Model file for the job. Use its own axes, mm. Face numbers are marked on the shaded views. A direction names the side the tool comes from. Give positions to 0.01 mm unless a question says otherwise; leave off trailing zeros. Loops run counter-clockwise (first coordinate to the right, second up) from the corner with the lowest first, then second, coordinate; pieces in that order, holes last. Notation, with made-up numbers: (-21, 4.25) - (13, 4.25) arc R17 ccw to (13, 9.25) - close; hole circle Ø8 at (8.25, -10). An arc over 180 degrees is marked (long way). Use a Markdown table: item, result.
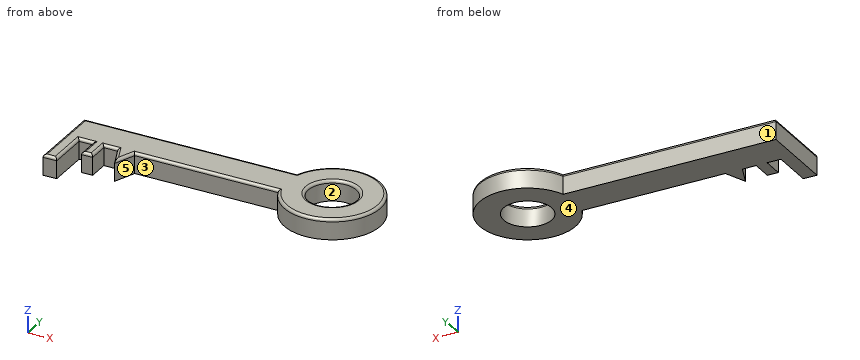
from build123d import *

# Parameters (mm, degrees)
F0_R     = 17.5
F0_W     = 10
F0_H     = 30
F0_W_2   = 8
F0_H_2   = 15
F1_DEPTH = 15
F2_R     = 2


with BuildPart() as f1:
    # F0 (on Top) → F1 (new body)
    with BuildSketch(Plane.XY):
        Polygon((70.049999, 32.850001), (-84.950001, 32.850001), (-84.950001, 7.850001), (-74.950001, 7.850001), (-64.950001, 7.850001), (-56.950001, 7.850001), (-46.950001, 7.850001), (-34.520773, 7.850001), (70.049999, 7.850001), align=None)
        with BuildLine():
            ThreePointArc((70.049999, 7.850001), (137.741741, 20.350001), (70.049999, 32.850001))
            Line((70.049999, 32.850001), (70.049999, 7.850001))
        make_face()
        with Locations((102.741741, 20.350001)):
            Circle(F0_R, mode=Mode.SUBTRACT)
        with Locations((-79.950001, -7.149999)):
            Rectangle(F0_W, F0_H)
        Polygon((-40.735387, -7.49211), (-34.520773, 7.850001), (-46.950001, 7.850001), align=None)
        with Locations((-60.950001, 0.350001)):
            Rectangle(F0_W_2, F0_H_2)
    extrude(amount=F1_DEPTH)

    # F2
    f2_edges = [f1.edges().sort_by_distance(p)[0] for p in [
        (-7.450001, 32.850001, 15),
        (-84.950001, 5.350001, 15),
        (-79.950001, -22.149999, 15),
        (-74.950001, -7.149999, 15),
        (-69.950001, 7.850001, 15),
        (-64.950001, 0.350001, 15),
        (-60.950001, -7.149999, 15),
        (-56.950001, 0.350001, 15),
        (-51.950001, 7.850001, 15),
        (-43.842694, 0.178945, 15),
        (-37.62808, 0.178945, 15),
        (17.764613, 7.850001, 15),
        (137.741741, 20.350001, 15),
        (85.241741, 20.350001, 15),
    ]]
    fillet(f2_edges, radius=F2_R)


solid = f1.part
(1) Slice it at A-A, the plane z = 8.5. Write the cut outline in (x, y).
Computed:
| item | result |
|---|---|
| outline | (-84.95, -22.15) - (-74.95, -22.15) - (-74.95, 7.85) - (-64.95, 7.85) - (-64.95, -7.15) - (-56.95, -7.15) - (-56.95, 7.85) - (-46.95, 7.85) - (-40.74, -7.49) - (-34.52, 7.85) - (70.05, 7.85) arc R35 ccw (long way) to (70.05, 32.85) - (-84.95, 32.85) - close; hole circle Ø35 at (102.74, 20.35) |
(2) Mould opens along X. For the marked faces 1, 2 and 3 say: pulls with the +X half, pulls with the -X half, needs draft (parallel to the pull), parting line crosses it, or undercut.
Computed:
| item | result |
|---|---|
| face 1 | needs draft |
| face 2 | undercut |
| face 3 | undercut |
(3) Slice it at B-B, the plane x = 34. Write the cut outline in (y, z).
Computed:
| item | result |
|---|---|
| outline | (7.85, 0) - (32.85, 0) - (32.85, 13) arc R2 ccw to (30.85, 15) - (9.85, 15) arc R2 ccw to (7.85, 13) - close |
(4) Pin check, flat tips, straight feed: P1, Ø1.5, axis at x = 89, z = 11.5, coming from the -Y side; P2, Ø5, axis at x = -71, z = 8.5, coming from the -Y side; P3, Ø2.5, axis at x = -62, z = 8, coming from the -Y side; P4, Ø21, axis at x = 102.74, y = 20.35, coming from the +Z side. Stop position of each tip, or through.
Computed:
| item | result |
|---|---|
| P1 | y = -12.15 |
| P2 | y = 7.85 |
| P3 | y = -7.15 |
| P4 | through |
(5) 3-axis set-ups, long thin cutter, end or side, ignore diameter. For the marked faces 4 and 5: which of +Z, -Z, +X, -X, +Y, -Y reach the whole face in a straight line?
Computed:
| item | result |
|---|---|
| face 4 | -Z, +X, -X, +Y, -Y |
| face 5 | +Z, -Z, -Y |
(6) Drill centre lines: probe 1 along X at (y, z) = (-7, 2.75); probe 2 along X at (y, z) = (-1, 2.5); probe 3 along Y at (x, z) = (-72, 1). Where is each one in solid material? Low to high. Write a range as [from, to].
Computed:
| item | result |
|---|---|
| probe 1 | [-84.95, -74.95], [-64.95, -56.95], [-40.93, -40.54], [80.9, 124.58] |
| probe 2 | [-84.95, -74.95], [-64.95, -56.95], [-43.37, -38.11], [75.01, 130.48] |
| probe 3 | [7.85, 32.85] |
